Geometry: see drawing. Coordinates: mm, zero at the bounding-box minimum. Coordinates: 2 decimals unless noted, no trailing zeros. Order: outer loops, then holes, each group sorted by start corner. A loop starts at its lowest first (then second) coordinate and runs counter-clockwise, first axis right, second up.
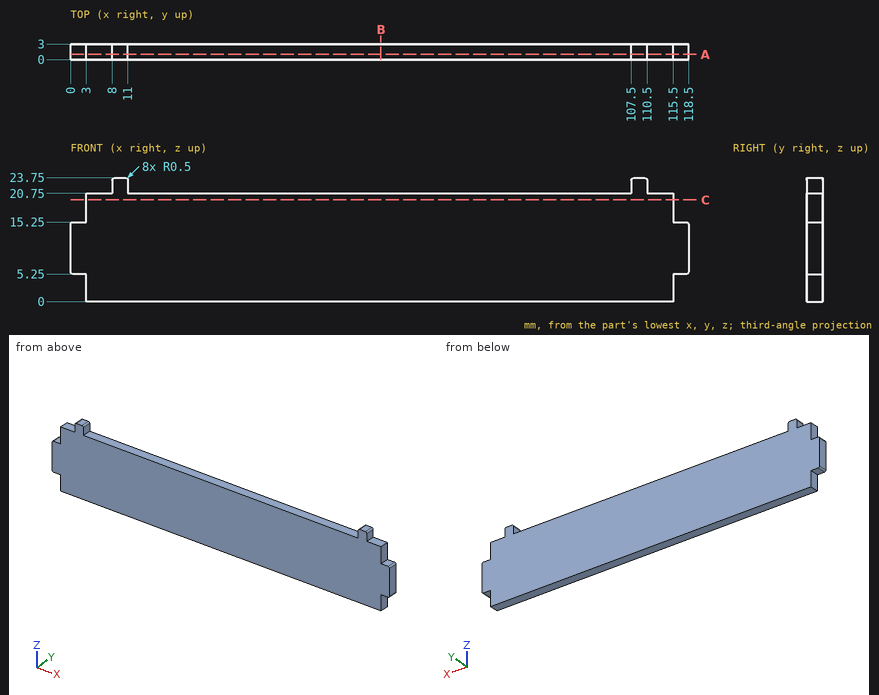
Q1. Section query B-B on x = 59.5. Output: boundary loops of the cut face in (y, z), plus the area to 4 significant figures.
Solutions:
outline: (0, 0) - (3, 0) - (3, 20.75) - (0, 20.75) - close
area: 62.25 mm2
Q2. Material intervals for line 1 along X through (y, z) = (1.8, 22); line 2 along Z through (x, y) = (77.5, 1.7); line 3 along X through (y, z) = (0.6, 18.5), sorted ascending.
Solutions:
line 1: x = 8 to 11, 107.5 to 110.5
line 2: z = 0 to 20.75
line 3: x = 3 to 115.5
Q3. Section query A-A on y = 1. Output: boundary loops of the cut face in (x, z), plus the area to 3 significant figures.
Solutions:
outline: (0, 5.75) arc R0.5 ccw to (0.5, 5.25) - (3, 5.25) - (3, 0) - (115.5, 0) - (115.5, 5.25) - (118, 5.25) arc R0.5 ccw to (118.5, 5.75) - (118.5, 14.75) arc R0.5 ccw to (118, 15.25) - (115.5, 15.25) - (115.5, 20.75) - (110.5, 20.75) - (110.5, 23.25) arc R0.5 ccw to (110, 23.75) - (108, 23.75) arc R0.5 ccw to (107.5, 23.25) - (107.5, 20.75) - (11, 20.75) - (11, 23.25) arc R0.5 ccw to (10.5, 23.75) - (8.5, 23.75) arc R0.5 ccw to (8, 23.25) - (8, 20.75) - (3, 20.75) - (3, 15.25) - (0.5, 15.25) arc R0.5 ccw to (0, 14.75) - close
area: 2,410 mm2
Q4. Section query C-C on z = 19.5. Output: boundary loops of the cut face in (x, y).
Solutions:
outline: (3, 0) - (115.5, 0) - (115.5, 3) - (3, 3) - close
Q5. Pin query (flat end, axial travel): P1, Ø0.9, axis at y = 1, z = 3.5, coming from the +X side; P2, Ø1.2, axis at y = 1.5, z = 21.5, coming from the +X side; P3, Ø1.5, axis at y = 2, z = 18, coming from the -X side. Return the tip coordinate at first contact, or that it passes through.
Solutions:
P1: stops at x = 115.5
P2: stops at x = 110.5
P3: stops at x = 3
